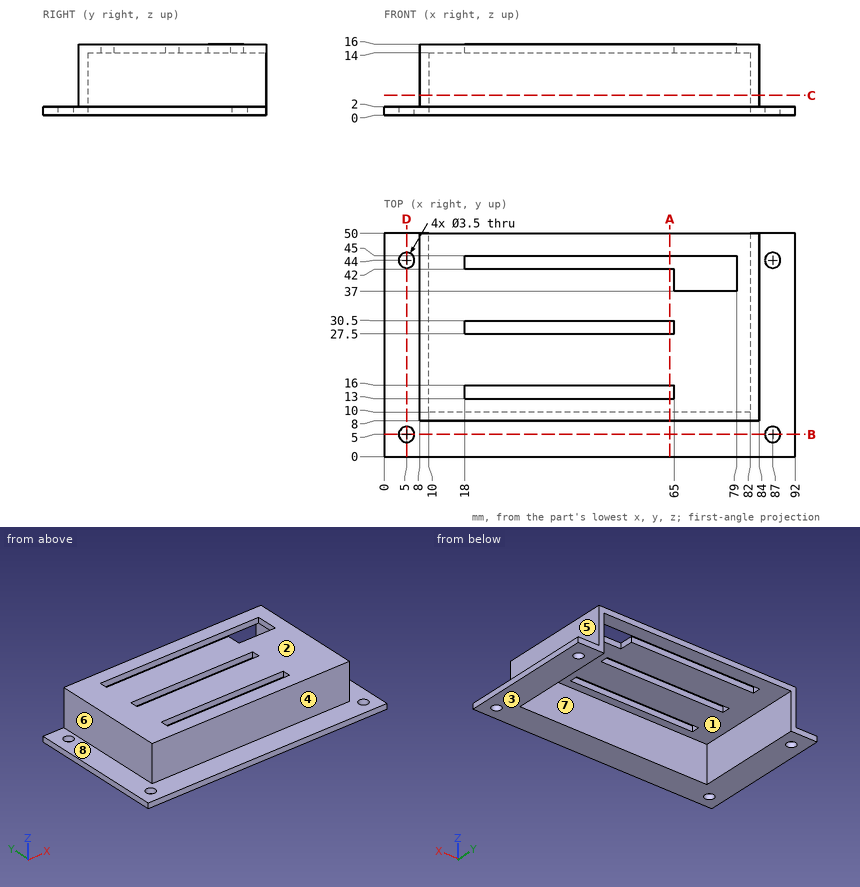
The drawing under review shows one solid part. Ordinate dimensions are in mm from its lowest x, y, z. A direction names the side the tool comes from. Coordinates: 2 decimals unless noted, no trailing zeros. Loops run counter-clockwise (first coordinate to the right, second up) from the corner with the lowest first, then second, coordinate; pieces in that order, holes last. Notation, with made-up numbers: M 62,58 L 87,58 A34 cw 87,94 Z; hole C 74.5,7 d11. An arc over 180 degrees is marked long. Use one line per item in the form item = value.
(1) For line 1 along X through (y, z) = (44, 0.85); line 2 along X through (y, z) = (5, 1.55); line 3 along Y through (x, z) = (87, 1.2), list the stretches that pass through material, from the lowest coordinate up. Write a range as from..to.
Return value:
line_1 = 0..3.25, 6.75..10, 82..85.25, 88.75..92
line_2 = 0..3.25, 6.75..85.25, 88.75..92
line_3 = 0..3.25, 6.75..42.25, 45.75..50
(2) For the marked faces 1, 2, 3, 4 and 5, list the 3-axis set-ups (+Z, -Z, +X, -X, +Y, -Y) from which the entire face can be reached by the end or side of a thin tool; tool diameter is ignored.
Return value:
face_1 = -Z, +Y
face_2 = +Z, +X, -X, +Y, -Y
face_3 = -Z, +X, -X, +Y, -Y
face_4 = +Z, +X, -X, -Y
face_5 = +Z, +X, +Y, -Y
(3) Consider section C-C (z = 4.5). Write out the cut boundary in (x, y), and give its area (3 significant figures).
Return value:
outline = M 8,8 L 84,8 L 84,50 L 82,50 L 82,10 L 10,10 L 10,50 L 8,50 Z
area = 312 mm2
(4) Clearance check with flat-ended pins moving along their axes: P1, Ø1, axis at y = 43, z = 15, coming from the +X side; P2, Ø1.5, axis at x = 72.5, z = 5.5, coming from the -Y side; P3, Ø10, axis at x = 16.5, y = 40.5, coming from the -Z side. State where each tip first meets the part, or that it passes through.
Return value:
P1 = 84
P2 = 8
P3 = 14
(5) Draft analysis for pull direction X (two halves, no side actions). For the marked faces 6, 7 and 8, state which applies: pulls with the +X half, pulls with the -X half, needs draft (parallel to the pull), parting line crosses it, or undercut.
Return value:
face_6 = pulls with the -X half
face_7 = undercut
face_8 = needs draft
(6) Consider section D-D (x = 5). Write out the cut boundary in (y, z), and give its area (3 significant figures).
Return value:
outline = M 0,0 L 3.25,0 L 3.25,2 L 0,2 Z; M 6.75,0 L 42.25,0 L 42.25,2 L 6.75,2 Z; M 45.75,0 L 50,0 L 50,2 L 45.75,2 Z
area = 86.0 mm2
(7) Consider section B-B (y = 5). Write out the cut boundary in (x, z), and give its area (3 significant figures).
Return value:
outline = M 0,0 L 3.25,0 L 3.25,2 L 0,2 Z; M 6.75,0 L 85.25,0 L 85.25,2 L 6.75,2 Z; M 88.75,0 L 92,0 L 92,2 L 88.75,2 Z
area = 170 mm2
(8) Consider section A-A (x = 64). Write out the cut boundary in (y, z), and give its area (3 significant figures).
Return value:
outline = M 0,0 L 10,0 L 10,14 L 13,14 L 13,16 L 8,16 L 8,2 L 0,2 Z; M 16,14 L 27.5,14 L 27.5,16 L 16,16 Z; M 30.5,14 L 42,14 L 42,16 L 30.5,16 Z; M 45,14 L 50,14 L 50,16 L 45,16 Z
area = 110 mm2
